Here's the drawing with two shaded views (mm, measured from the low corner). I have some questions. A direction names the side the tool comes from. Give positions to 0.01 mm unless a question says otherwise; leave off trailing zeros. Loops run counter-clockwise (first coordinate to the right, second up) from the corner with the lowest first, then second, coordinate; pieces in that order, holes last. Notation, with made-up numbers: M -23,36 L -12,36 A23 cw -12,66 Z; hole C 30.25,41.25 d7. An arc over 180 degrees is marked long. Put each result on its own line as item: value. Start each with the question number.
1) Imagine slicing it at A-A (z = 24.5). Write out the boundary of the cut face in (x, y), then the cut area to 3 significant figures.
2) For P1, Ø3, axis at y = 32.5, z = 46.5, coming from the -X side; P2, Ø1, axis at y = 11, z = 36, coming from the -X side; P3, Ø14, axis at y = 7, z = 22, coming from the +X side; P4, Ø6, axis at y = 18.5, z = 37, coming from the -X side, each with a flat end and sliding along its axis, tell me the tip position at first contact or that it passes through.
3) Imagine slicing it at C-C (x = 11). Write out the boundary of the cut face in (y, z).
4) Imagine slicing it at D-D (y = 20). Write out the boundary of the cut face in (x, z).
5) Imagine slicing it at B-B (x = 21.5). Write out the boundary of the cut face in (y, z).
6) If we mould it in two halves opening along Y, with no side actions, what happens to the marked faces 6, 7 and 8? For each: +Y half, -Y half, draft (parallel to the pull), parting line (faces both ways), or undercut.
7) For the marked faces 1, 2, 3, 4 and 5, which set-ups out of +Z, -Z, +X, -X, +Y, -Y let a thin tool reach every point of the face, with its end or its side?
8) Please list where these lines run through material, in increasing order: line 1 along Y through (x, z) = (22, 24); line 2 along Z through (x, y) = (6.5, 22.5); line 3 along X through (y, z) = (46, 16). Write a range as from..to.
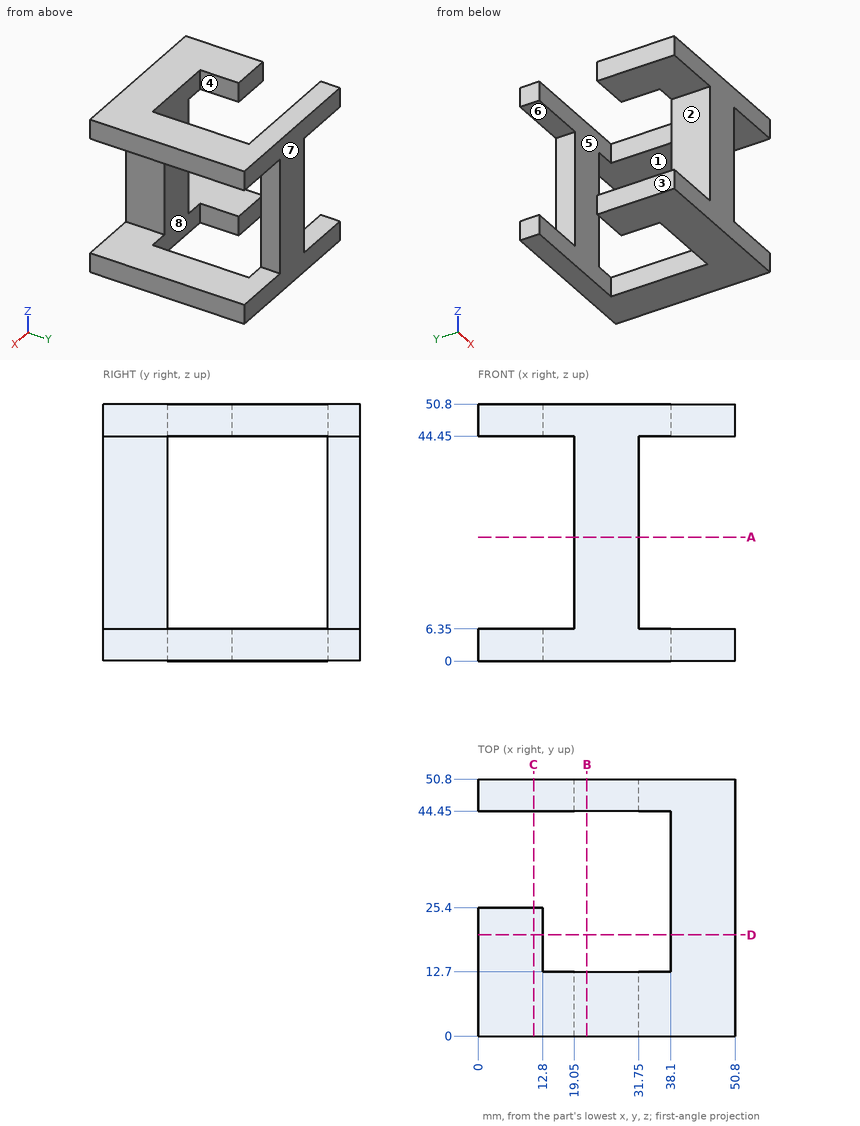
Recorded:
1. outline: M 19.05,0 L 31.75,0 L 31.75,12.7 L 19.05,12.7 Z; M 19.05,44.45 L 31.75,44.45 L 31.75,50.8 L 19.05,50.8 Z
1. area: 242 mm²
2. P1: x = 38.1
2. P2: x = 19.05
2. P3: x = 31.75
2. P4: through
3. outline: M 0,0 L 25.4,0 L 25.4,6.35 L 0,6.35 Z; M 0,44.45 L 25.4,44.45 L 25.4,50.8 L 0,50.8 Z; M 44.45,0 L 50.8,0 L 50.8,6.35 L 44.45,6.35 Z; M 44.45,44.45 L 50.8,44.45 L 50.8,50.8 L 44.45,50.8 Z
4. outline: M 0,0 L 12.8,0 L 12.8,6.35 L 0,6.35 Z; M 0,44.45 L 12.8,44.45 L 12.8,50.8 L 0,50.8 Z; M 38.1,0 L 50.8,0 L 50.8,6.35 L 38.1,6.35 Z; M 38.1,44.45 L 50.8,44.45 L 50.8,50.8 L 38.1,50.8 Z
5. outline: M 0,0 L 12.7,0 L 12.7,50.8 L 0,50.8 Z; M 44.45,0 L 50.8,0 L 50.8,50.8 L 44.45,50.8 Z
6. face 6: draft
6. face 7: +Y half
6. face 8: undercut
7. face 1: +X, +Y, -Y
7. face 2: -X, +Y, -Y
7. face 3: +Z, -Z, -X, +Y, -Y
7. face 4: +Z, -Z
7. face 5: +Z, -Z, -X
8. line 1: 0..12.7, 44.45..50.8
8. line 2: 0..6.35, 44.45..50.8
8. line 3: 19.05..31.75
